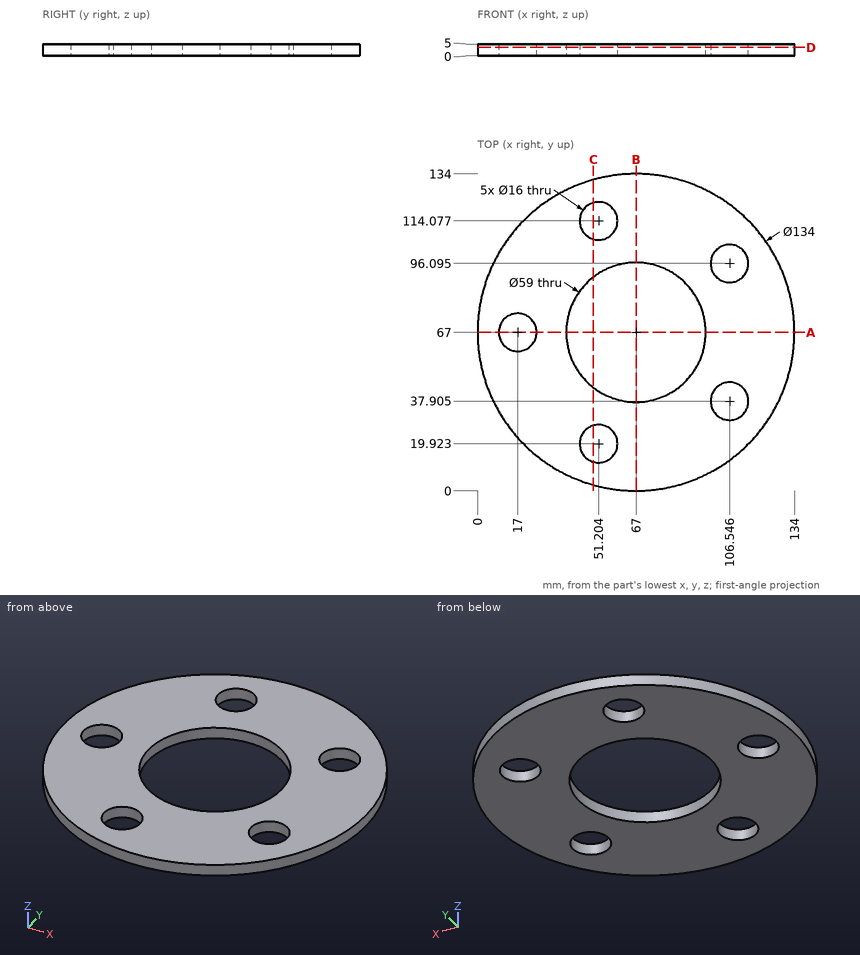
Study the drawing (mm; zero at the part's minimum x, y, z) and answer. Round coordinates to 2 decimals unless told otherwise and drop trailing zeros. Order: outer loops, then holes, each group sorted by start corner. A loop starts at its lowest first (then second) coordinate and runs counter-clockwise, first axis right, second up. Notation, with made-up numbers: (-13.75, 8.5) - (18.25, 8.5) arc R15 ccw to (18.25, 23.5) - close; hole circle Ø3 at (80.5, 88.5). An arc over 180 degrees is marked (long way). Use one line per item in the form item = value. Start each with the question number.
(1) The part is cut by section B-B (x = 67). Give the vertices of the cut face in (y, z).
(2) Flat-ended cylindrical pins translate along their axes: pin 1 Ø2 at (y, z) = (32, 2.5) entering from +X; pin 2 Ø3 at (x, z) = (108, 3) entering from -Y. Find the tip coordinate at first contact, or state that the pin passes through.
(3) The part is cut by section A-A (y = 67). Give the vertices of the cut face in (x, z).
(4) Find the intervals of material crossed by line 1 along Y through (x, z) = (67, 3.65); line 2 along X through (y, z) = (91, 1.95) (1 decimal); line 3 along Y through (x, z) = (107, 2.3), in increasing order. Write a range as from..to.
(5) The part is cut by section D-D (z = 3.55). Give the vertices of the cut face in (x, y) (1 decimal).
(6) The part is cut by section C-C (x = 49). Give the vertices of the cut face in (y, z).
Checked values:
q1.outline = (0, 0) - (37.5, 0) - (37.5, 5) - (0, 5) - close; (96.5, 0) - (134, 0) - (134, 5) - (96.5, 5) - close
q2.pin_1 = 124.73
q2.pin_2 = 12.88
q3.outline = (0, 0) - (9, 0) - (9, 5) - (0, 5) - close; (25, 0) - (37.5, 0) - (37.5, 5) - (25, 5) - close; (96.5, 0) - (134, 0) - (134, 5) - (96.5, 5) - close
q4.line_1 = 0..37.5, 96.5..134
q4.line_2 = 4.4..49.8, 84.2..100.4, 112.7..129.6
q4.line_3 = 13.25..29.92, 45.89..88.11, 104.08..120.75
q5.outline = circle Ø134 at (67, 67); hole circle Ø16 at (17, 67); hole circle Ø59 at (67, 67); hole circle Ø16 at (51.2, 19.9); hole circle Ø16 at (51.2, 114.1); hole circle Ø16 at (106.5, 37.9); hole circle Ø16 at (106.5, 96.1)
q6.outline = (2.46, 0) - (12.23, 0) - (12.23, 5) - (2.46, 5) - close; (27.61, 0) - (43.63, 0) - (43.63, 5) - (27.61, 5) - close; (90.37, 0) - (106.39, 0) - (106.39, 5) - (90.37, 5) - close; (121.77, 0) - (131.54, 0) - (131.54, 5) - (121.77, 5) - close
